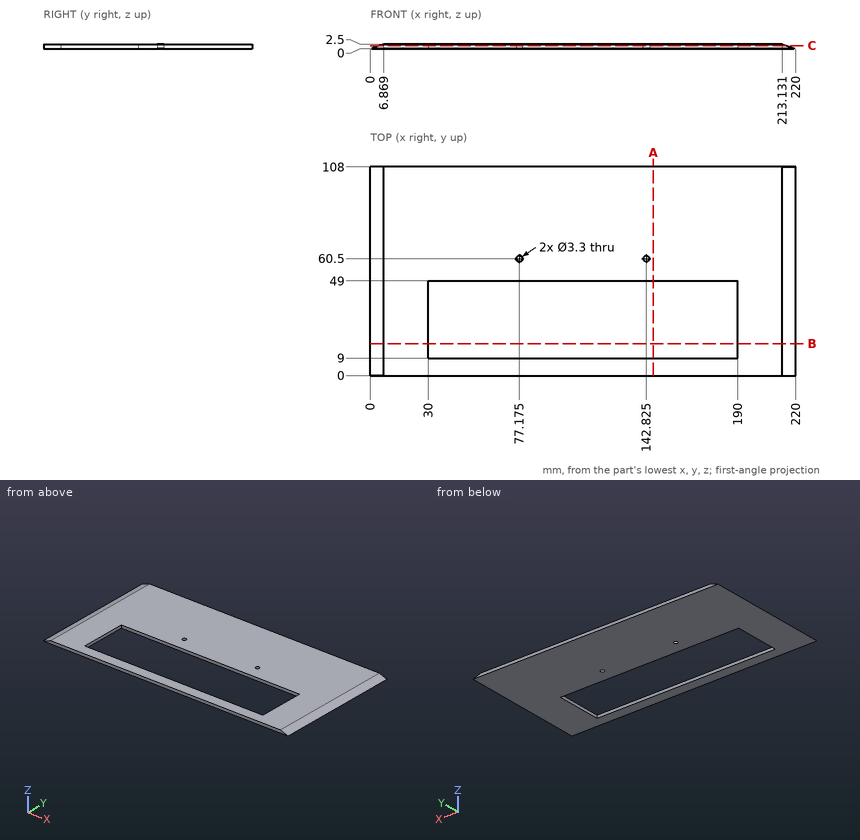
Answer from the drawing. Dimensions are ordinates in mm from the lowest x, y and z of the part. Give positions to 0.01 mm unless a question says otherwise; leave off trailing zeros. Order: outer loops, then holes, each group sorted by start corner. A loop starts at its lowest first (then second) coordinate and runs counter-clockwise, first axis right, second up. Notation, with made-up numbers: (87, 74.25) - (103, 74.25) arc R20 ccw to (103, 83.25) - close; hole circle Ø2 at (27.25, -37.5). An arc over 180 degrees is marked (long way). One line per item, written item: value. Start each with the question number.
1. Section C-C, the plane z = 1.65 is taken. Count the separate pieces of the cut face and the enclosed holes in it, then the cut area to 3 significant figures.
2. This flat-tipped pin is pushed along its axis until it touches: pin 1 Ø4 at (x, y) = (180.5, 12) entering from -Z. Where does it stop, or does it pass through?
3. Consider line 1 (Y direction, x = 107, z = 0.9). Determine where the line is inside the solid, lowest interval first.
4. Section B-B, the plane y = 16.5 is taken. Write down the section's boundary in (x, z).
5. Section A-A, the plane x = 146.5 is taken. Write down the section's boundary in (y, z), then the cut area to 3 significant figures.
Filled sheet:
1. separate pieces: 1
1. enclosed holes: 3
1. area: 16,400 mm²
2. pin 1: through
3. line 1: 0 to 9, 49 to 108
4. outline: (0, 0) - (30, 0) - (30, 2.5) - (6.87, 2.5) - close; (190, 0) - (220, 0) - (213.13, 2.5) - (190, 2.5) - close
5. outline: (0, 0) - (9, 0) - (9, 2.5) - (0, 2.5) - close; (49, 0) - (108, 0) - (108, 2.5) - (49, 2.5) - close
5. area: 170 mm²
